```python
from build123d import *

# Parameters (mm, degrees)
F0_W      = 120
F0_H      = 15
F1_DEPTH  = 40
F2_W      = 60
F2_H      = 5
F3_DEPTH  = 80.001
F4_R      = 5
F5_DEPTH  = 15.001
F6_R      = 35
F6_R_2    = 25
F7_DEPTH  = 30
F9_DEPTH  = 30
F11_DEPTH = 10


with BuildPart() as f1:
    # F0 (on Front) → F1 (new body, symmetric)
    with BuildSketch(Plane.XZ):
        Rectangle(F0_W, F0_H)
    extrude(amount=F1_DEPTH, both=True)

    # F2 (on face) → F3 (cut, through all)
    with BuildSketch(Plane.XZ.offset(40)):
        with Locations((-2.0098921657, -5)):
            Rectangle(F2_W, F2_H)
    extrude(amount=-F3_DEPTH, mode=Mode.SUBTRACT)

    # F4 (on face) → F5 (cut, through all)
    with BuildSketch(Plane.XY.offset(7.5)):
        with Locations((-45, 25)):
            Circle(F4_R)
        with Locations((-45, -25)):
            Circle(F4_R)
        with Locations((45, -25)):
            Circle(F4_R)
        with Locations((45, 25)):
            Circle(F4_R)
    extrude(amount=-F5_DEPTH, mode=Mode.SUBTRACT)



with BuildPart() as f7:
    # F6 (on Front) → F7 (new body, symmetric)
    with BuildSketch(Plane.XZ):
        with Locations((30, 67.5)):
            Circle(F6_R)
        with Locations((30, 67.5)):
            Circle(F6_R_2, mode=Mode.SUBTRACT)
    extrude(amount=F7_DEPTH, both=True)


with BuildPart() as f1_1:
    add(f1.part)

    add(f7.part)  # F9 merges F7
    # F8 (on Front) → F9 (join)
    with BuildSketch(Plane.XZ):
        with BuildLine():
            ThreePointArc((35, 32.8589838486), (30, 32.5), (25, 32.8589838486))
            Line((25, 32.8589838486), (25, 7.5))
            Line((25, 7.5), (35, 7.5))
            Line((35, 7.5), (35, 32.8589838486))
        make_face()
    extrude(amount=F9_DEPTH)

    # F10 (on Front) → F11 (join)
    with BuildSketch(Plane.XZ):
        with BuildLine():
            ThreePointArc((25, 32.8589838486), (2.2005780667, 46.2351900979), (-4.7421322486, 71.740783751))
            Line((-4.7421322486, 71.740783751), (-25, 7.5))
            Line((-25, 7.5), (25, 7.5))
            Line((25, 7.5), (25, 32.8589838486))
        make_face()
    extrude(amount=F11_DEPTH)


solid = f1_1.part
```
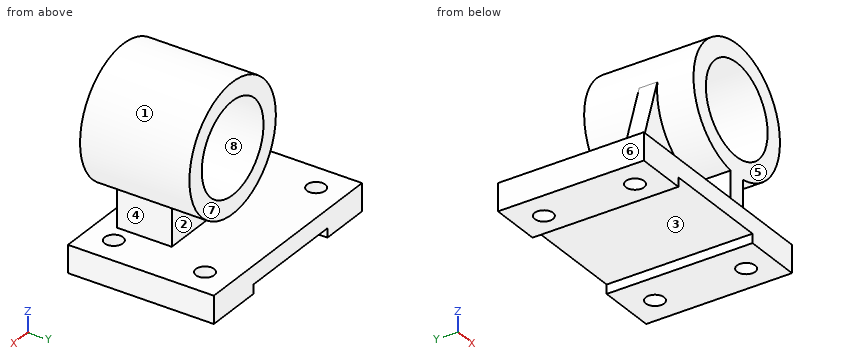
Can you work these out from the model? Positions are in its coordinate system, mm. Face numbers are marked on the shaded views. A direction names the side the tool comes from. Coordinates: 2 decimals unless noted, no trailing zeros. Order: outer loops, then holes, each group sorted by start corner. A loop starts at its lowest first (then second) coordinate and runs counter-clockwise, first axis right, second up.
1. If we section it at C-C (x = 30): Please give me the cut outline in (y, z).
2. If we section it at B-B (y = 9.5): Please give me the cut outline in (x, z).
3. If we section it at D-D (z = 1): Please give me the cut outline in (x, y).
4. Thinking about a two-plate mould opening in X: for the marked faces 6, 7 and 8, which applies, +X half, -X half, draft (parallel to the pull), parting line (faces both ways), or undercut?
5. If we section it at A-A (y = 25): Please give me the cut outline in (x, z).
6. I need wall thicknesses on line 1 (Y direction, x = -45, z = -3.5); line 2 (Z direction, x = 38.5, y = -5); line 3 (Z direction, x = 38, y = -0.5). Which ranges of each line are inside material? Lowest first, please.
7. For the marked faces 1, 2, 3, 4 and 5, which set-ups out of +Z, -Z, +X, -X, +Y, -Y let a thin tool reach every point of the face, with its end or its side?
8. I'm going to push flat-ended pins straight in: pin 1 (20.5 mm diameter, centred on y = -14, z = 22.5, fed in from +X); pin 2 (5 mm diameter, centred on x = 18.5, z = 14, fed in from -Y); pin 3 (11.5 mm diameter, centred on x = 45, y = 25, fed in from +Z). Where does each tip first touch, or does it pass through?
Entries:
1. outline: (-40, -7.5) - (40, -7.5) - (40, 7.5) - (0, 7.5) - (0, 32.5) - (30, 32.5) - (30, 42.5) - (-30, 42.5) - (-30, 7.5) - (-40, 7.5) - close; (-30, 92.5) - (30, 92.5) - (30, 102.5) - (-30, 102.5) - close
2. outline: (-60, -7.5) - (-32.01, -7.5) - (-32.01, -2.5) - (27.99, -2.5) - (27.99, -7.5) - (60, -7.5) - (60, 7.5) - (-60, 7.5) - close; circle Ø70 at (30, 67.5); hole circle Ø50 at (30, 67.5)
3. outline: (-60, -40) - (60, -40) - (60, 40) - (-60, 40) - close; hole circle Ø10 at (-45, -25); hole circle Ø10 at (-45, 25); hole circle Ø10 at (45, -25); hole circle Ø10 at (45, 25)
4. face 6: -X half
4. face 7: draft
4. face 8: undercut
5. outline: (-60, -7.5) - (-50, -7.5) - (-50, 7.5) - (-60, 7.5) - close; (-40, -7.5) - (-32.01, -7.5) - (-32.01, -2.5) - (27.99, -2.5) - (27.99, -7.5) - (40, -7.5) - (40, 7.5) - (-40, 7.5) - close; circle Ø70 at (30, 67.5); (50, -7.5) - (60, -7.5) - (60, 7.5) - (50, 7.5) - close; hole circle Ø50 at (30, 67.5)
6. line 1: y = -40 to -30, -20 to 20, 30 to 40
6. line 2: z = -7.5 to 7.5, 33.55 to 43.99, 91.01 to 101.45
6. line 3: z = -7.5 to 7.5, 33.43 to 43.81, 91.19 to 101.57
7. face 1: none
7. face 2: -X, +Y
7. face 3: -Z, +Y, -Y
7. face 4: +X, +Y, -Y
7. face 5: +Z, +X, -X, -Y
8. pin 1: stops at x = 35
8. pin 2: stops at y = -10
8. pin 3: stops at z = 101.26
